```python
from build123d import *

# Parameters (mm, degrees)
SKETCH1_W           = 6.5
SKETCH1_H           = 6.5
BOSS_EXTRUDE1_DEPTH = 2
SKETCH2_R           = 1.5
BOSS_EXTRUDE2_DEPTH = 1
FILLET1_R           = 0.1
FILLET2_R           = 0.05
BOSS_EXTRUDE3_DEPTH = 6.5
SKETCH4_W           = 2
SKETCH4_H           = 1.55
SKETCH4_H_2         = 4.1
SKETCH4_H_3         = 0.2
CUT_EXTRUDE1_DEPTH  = 4


with BuildPart() as part:
    # Sketch1 → Boss-Extrude1 (new body)
    with BuildSketch(Plane(origin=(0, 0, 0), x_dir=(1, 0, 0), z_dir=(0, 1, 0))):
        with Locations((3.25, 3.25)):
            Rectangle(SKETCH1_W, SKETCH1_H)
    extrude(amount=BOSS_EXTRUDE1_DEPTH)

    # Sketch2 → Boss-Extrude2 (add)
    with BuildSketch(Plane(origin=(0, 2, 0), x_dir=(1, 0, 0), z_dir=(0, 1, 0))):
        with Locations((3.25, 3.25)):
            Circle(SKETCH2_R)
    extrude(amount=BOSS_EXTRUDE2_DEPTH)

    # Fillet1
    fillet1_edges = [part.edges().sort_by_distance(p)[0] for p in [
        (1.75, 3, -3.25),
    ]]
    fillet(fillet1_edges, radius=FILLET1_R)

    # Fillet2
    fillet2_edges = [part.edges().sort_by_distance(p)[0] for p in [
        (6.5, 2, -3.25),
        (3.25, 2, -6.5),
        (0, 2, -3.25),
        (3.25, 2, 0),
    ]]
    fillet(fillet2_edges, radius=FILLET2_R)

    # Sketch3 → Boss-Extrude3 (add, through all)
    with BuildSketch(Plane.XY):
        Polygon((6.5, 1), (7.566666667, 0.2), (8.5, 0.2), (8.5, 0), (7.5, 0), (6.5, 0.75), align=None)
        Polygon((-2, 0), (-1, 0), (0, 0.75), (0, 1), (-1.066666667, 0.2), (-2, 0.2), align=None)
    extrude(amount=-BOSS_EXTRUDE3_DEPTH)

    # Sketch4 → Cut-Extrude1 (cut, through all)
    with BuildSketch(Plane(origin=(0, 0, 0), x_dir=(-1, 0, 0), z_dir=(0, -1, 0))):
        with Locations((1, 1.975)):
            Rectangle(SKETCH4_W, SKETCH4_H)
        with Locations((1, 4.525)):
            Rectangle(SKETCH4_W, SKETCH4_H)
        with Locations((-7.5, 3.25)):
            Rectangle(SKETCH4_W, SKETCH4_H_2)
        with Locations((1, 0.1)):
            Rectangle(SKETCH4_W, SKETCH4_H_3)
        with Locations((1, 6.4)):
            Rectangle(SKETCH4_W, SKETCH4_H_3)
        with Locations((-7.5, 6.4)):
            Rectangle(SKETCH4_W, SKETCH4_H_3)
        with Locations((-7.5, 0.1)):
            Rectangle(SKETCH4_W, SKETCH4_H_3)
    extrude(amount=-CUT_EXTRUDE1_DEPTH, mode=Mode.SUBTRACT)


solid = part.part
```
The listing builds one solid part. Answer for the finished solid, in the listing's coordinates (mm). A direction names the side the tool comes from. Coordinates: 2 decimals unless noted, no trailing zeros. Loops run counter-clockwise (first coordinate to the right, second up) from the corner with the lowest first, then second, coordinate; pieces in that order, holes last. Notation, with made-up numbers: (9.5, 20) - (59.5, 20) arc R16 ccw to (59.5, 33) - close; hole circle Ø1 at (23, 27). An arc over 180 degrees is marked (long way). Use a Markdown table: item, result. Add a question column.
1) The part is cut by section A-A, the plane x = -0.25. Give the vertices of the cut face in (y, z).
2) The part is cut by section C-C, the plane y = 0.35. Give the vertices of the cut face in (x, z), and give its area (3 significant figures).
3) The part is cut by section B-B, the plane z = -6. Give the vertices of the cut face in (x, y).
4) For faces 1 (the flat face through (5, 2, -4)), 2 (the flat face through (8, 0.2, -6)), 3 (the flat face through (-1.5, 0.2, -0.7)), determine the directions among +Z, -Z, +X, -X, +Y, -Y from which every point of the face is accessible in a straight line to the end or side of a thin tool.
5) The part is cut by section D-D, the plane x = 3.25. Give the vertices of the cut face in (y, z).
6) Given pin 1 (1.1 mm diameter, centred on x = 8, y = 0.5, fed in from +Z); pin 2 (1 mm diameter, centred on x = -1.5, z = -3, fed in from +Y); pin 3 (1.5 mm diameter, centred on x = 7.5, y = 0.5, fed in from -Z), each flat-ended and moving along its own axis, determine where each tip first touches the part or whether it passes through.
7) Find the intervals of material crossed by line 1 (X direction, y = 0.55, z = -2.25); line 2 (Y direction, x = 3.75, z = -6); line 3 (X direction, y = 2.4, z = -4.5), in increasing order.
Here are the results:
| question | item | result |
|---|---|---|
| 1 | outline | (0.56, -6.3) - (0.81, -6.3) - (0.81, -5.3) - (0.56, -5.3) - close; (0.56, -3.75) - (0.81, -3.75) - (0.81, -2.75) - (0.56, -2.75) - close; (0.56, -1.2) - (0.81, -1.2) - (0.81, -0.2) - (0.56, -0.2) - close |
| 2 | outline | (-0.87, -6.3) - (-0.53, -6.3) - (-0.53, -5.3) - (-0.87, -5.3) - close; (-0.87, -3.75) - (-0.53, -3.75) - (-0.53, -2.75) - (-0.87, -2.75) - close; (-0.87, -1.2) - (-0.53, -1.2) - (-0.53, -0.2) - (-0.87, -0.2) - close; (0, -6.5) - (6.5, -6.5) - (6.5, 0) - (0, 0) - close; (7.03, -6.3) - (7.37, -6.3) - (7.37, -5.3) - (7.03, -5.3) - close; (7.03, -1.2) - (7.37, -1.2) - (7.37, -0.2) - (7.03, -0.2) - close |
| 2 | area | 43.9 mm^2 |
| 3 | outline | (-2, 0) - (-1, 0) - (0, 0.75) - (0, 0) - (6.5, 0) - (6.5, 0.75) - (7.5, 0) - (8.5, 0) - (8.5, 0.2) - (7.57, 0.2) - (6.5, 1) - (6.5, 1.95) arc R0.05 ccw to (6.45, 2) - (0.05, 2) arc R0.05 ccw to (0, 1.95) - (0, 1) - (-1.07, 0.2) - (-2, 0.2) - close |
| 4 | face 1 | +Y |
| 4 | face 2 | +Z, -Z, +X, +Y |
| 4 | face 3 | +Z, -Z, -X, +Y |
| 5 | outline | (0, -6.5) - (1.95, -6.5) arc R0.05 ccw to (2, -6.45) - (2, -4.75) - (2.9, -4.75) arc R0.1 ccw to (3, -4.65) - (3, -1.85) arc R0.1 ccw to (2.9, -1.75) - (2, -1.75) - (2, -0.05) arc R0.05 ccw to (1.95, 0) - (0, 0) - close |
| 6 | pin 1 | stops at z = -0.2 |
| 6 | pin 2 | stops at y = 0.25 |
| 6 | pin 3 | stops at z = -6.3 |
| 7 | line 1 | x = 0 to 6.5 |
| 7 | line 2 | y = 0 to 2 |
| 7 | line 3 | x = 2.42 to 4.08 |
